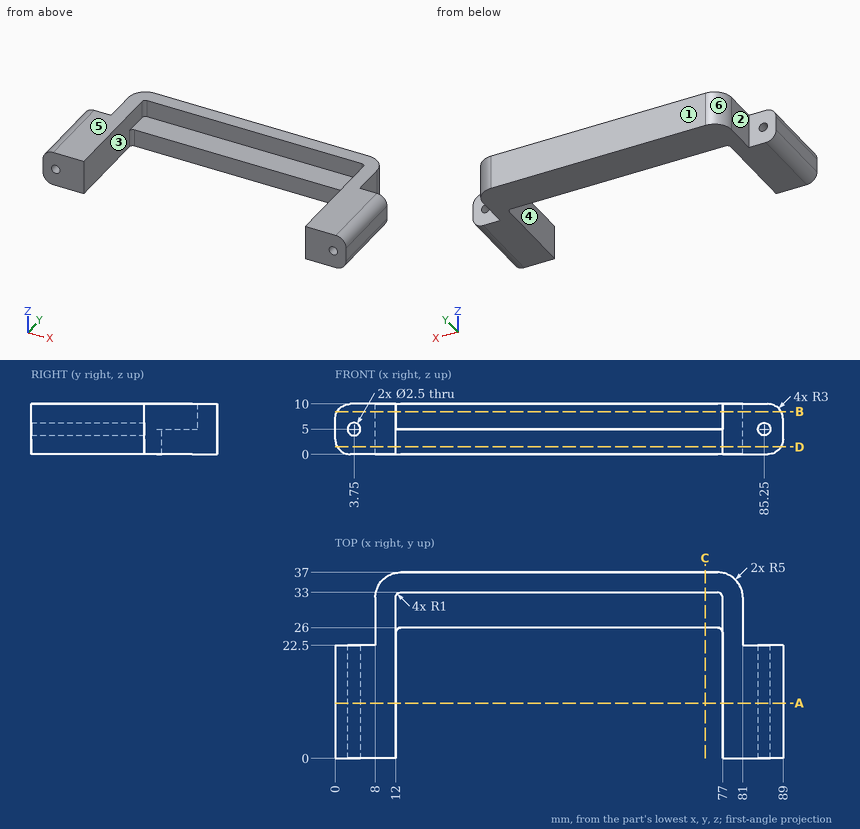
Could you check a few things on this drawing? It's one solid part, dimensions in mm from its lowest x, y, z. A direction names the side the tool comes from. Round coordinates to 2 decimals unless told otherwise and drop trailing zeros. Order: outer loops, then holes, each group sorted by start corner. A loop starts at its lowest first (then second) coordinate and runs counter-clockwise, first axis right, second up. Notation, with made-up numbers: M 50,57 L 57,57 A27 ccw 57,92 Z; hole C -10.75,-17.75 d11. An arc over 180 degrees is marked long. Return JSON: item names as keys, results as strings. Group by question number.
1. If we section it at D-D on z = 1.5: List the corners of the cut face in (x, y) for me.
2. I'm going to push flat-ended pins straight in: pin 1 Ø1 at (y, z) = (31.5, 2.5) entering from -X; pin 2 Ø1 at (x, z) = (46, 9) entering from -Y; pin 3 Ø2 at (x, z) = (3.75, 5) entering from +Y; pin 4 Ø5.5 at (x, z) = (48, 2) entering from -Y. Where does each tip first touch, or does it pass through?
3. On a 3-axis mill with a long thin cutter (end or side, diameter ignored), from which of +Z, -Z, +X, -X, +Y, -Y can I reach the whole of each face in a straight line? I mean the marked faces 1 and 2. Say none if no direction works.
4. If we section it at B-B on z = 8.5: List the corners of the cut face in (x, y) for me, then the cut area to 3 significant figures.
5. If we mould it in two halves opening along X, with no side actions, what happens to the marked faces 3, 4, 5 and 6? For each: pulls with the +X half, pulls with the -X half, needs draft (parallel to the pull), parting line crosses it, or undercut.
6. Please list where these lines run through material, in increasing order: probe 1 along Z at (x, y) = (85.25, 4.75); probe 2 along X at (y, z) = (5, 7); probe 3 along Y at (x, z) = (64, 1).
7. If we section it at A-A on y = 11: List the corners of the cut face in (x, z) for me.
8. If we section it at C-C on x = 73.5: List the corners of the cut face in (y, z) for me.
Reply:
{
 "1": {"outline": "M 0.4,0 L 12,0 L 12,25 A1 cw 13,26 L 76,26 A1 cw 77,25 L 77,0 L 88.6,0 L 88.6,22.5 L 81,22.5 L 81,32 A5 ccw 76,37 L 13,37 A5 ccw 8,32 L 8,22.5 L 0.4,22.5 Z"},
 "2": {"pin 1": "x = 8", "pin 2": "y = 33", "pin 3": "through", "pin 4": "y = 26"},
 "3": {"face 1": "+Z, -Z, +X, -X, +Y", "face 2": "+Z, -Z, -X, +Y"},
 "4": {"outline": "M 0.4,0 L 12,0 L 12,32 A1 cw 13,33 L 76,33 A1 cw 77,32 L 77,0 L 88.6,0 L 88.6,22.5 L 81,22.5 L 81,32 A5 ccw 76,37 L 13,37 A5 ccw 8,32 L 8,22.5 L 0.4,22.5 Z", "area": "888 mm^2"},
 "5": {"face 3": "undercut", "face 4": "undercut", "face 5": "needs draft", "face 6": "pulls with the -X half"},
 "6": {"probe 1": "0 to 3.75, 6.25 to 10", "probe 2": "0 to 12, 77 to 89", "probe 3": "26 to 37"},
 "7": {"outline": "M 0,3 A3 ccw 3,0 L 12,0 L 12,10 L 3,10 A3 ccw 0,7 Z; M 77,0 L 86,0 A3 ccw 89,3 L 89,7 A3 ccw 86,10 L 77,10 Z; hole C 3.75,5 d2.5; hole C 85.25,5 d2.5"},
 "8": {"outline": "M 26,0 L 37,0 L 37,10 L 33,10 L 33,5 L 26,5 Z"}
}
